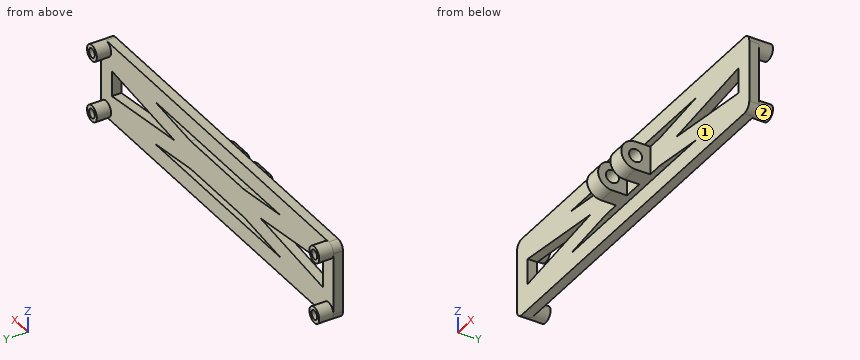
```python
from build123d import *

# Parameters (mm, degrees)
SKETCH2_W               = 80.1
SKETCH2_H               = 16.45
SKETCH2_W_2             = 72.76
SKETCH2_H_2             = 9.11
EXTRUDE_THIN1_DEPTH     = 2
EXTRUDE_THIN2_DEPTH     = 2
SKETCH6_W               = 18.3804486
SKETCH6_H               = 6
BOSS_EXTRUDE2_DEPTH     = 2
SKETCH7_R               = 1.375
BOSS_EXTRUDE3_DEPTH     = 3.8
LPATTERN1_COUNT         = 2
LPATTERN1_PITCH         = 8
FILLET2_R               = 1.69
SKETCH8_R               = 1.69
BOSS_EXTRUDE4_DEPTH     = 3
CUT_EXTRUDE1_START      = 3
SKETCH4_R               = 0.985
CUT_EXTRUDE1_DEPTH      = 4
MIRROR2_COPY_1_SKETCH_R = 1.69
MIRROR2_COPY_1_DEPTH    = 3
MIRROR2_START           = 3
MIRROR2_COPY_2_SKETCH_R = 0.985
MIRROR2_COPY_2_DEPTH    = 4


with BuildPart() as part:
    # Sketch2 → Extrude-Thin1 (new body)
    with BuildSketch(Plane(origin=(0, 0, 0), x_dir=(1, 0, 0), z_dir=(0, 1, 0))):
        Rectangle(SKETCH2_W, SKETCH2_H)
        Rectangle(SKETCH2_W_2, SKETCH2_H_2, mode=Mode.SUBTRACT)
    extrude(amount=EXTRUDE_THIN1_DEPTH)

    # Sketch3 → Extrude-Thin2 (add, through all)
    with BuildSketch(Plane(origin=(0, 2, 0), x_dir=(1, 0, 0), z_dir=(0, 1, 0))):
        Polygon((-36.607973326, 2.734216333), (36.152026674, -6.375783667), (36.607973326, -2.734216333), (-36.152026674, 6.375783667), align=None)
        Polygon((36.152026674, 6.375783667), (-36.607973326, -2.734216333), (-36.152026674, -6.375783667), (36.607973326, 2.734216333), align=None)
    extrude(amount=-EXTRUDE_THIN2_DEPTH)

    # Sketch6 → Boss-Extrude2 (add, through all)
    with BuildSketch(Plane(origin=(0, 2, 0), x_dir=(1, 0, 0), z_dir=(0, 1, 0))):
        Rectangle(SKETCH6_W, SKETCH6_H)
    extrude(amount=-BOSS_EXTRUDE2_DEPTH)

    # Sketch7 → Boss-Extrude3 (add)
    with BuildSketch(Plane(origin=(5.9, 0, 0), x_dir=(0, 0, -1), z_dir=(1, 0, 0))):
        with BuildLine():
            Line((-3, -3.1), (-3, 0))
            Line((-3, 0), (3, 0))
            Line((3, 0), (3, -3.1))
            ThreePointArc((3, -3.1), (0, -6.1), (-3, -3.1))
        make_face()
        with Locations((0, -3.1)):
            Circle(SKETCH7_R, mode=Mode.SUBTRACT)
    boss_extrude3 = extrude(amount=-BOSS_EXTRUDE3_DEPTH)

    # LPattern1: Boss-Extrude3 ×2
    with Locations(*[(-i * LPATTERN1_PITCH, 0, 0) for i in range(1, LPATTERN1_COUNT)]):
        add(boss_extrude3)

    # Fillet2
    fillet2_edges = [part.edges().sort_by_distance(p)[0] for p in [
        (40.05, 1, 8.225),
        (-40.05, 1, 8.225),
        (-40.05, 1, -8.225),
        (40.05, 1, -8.225),
    ]]
    fillet(fillet2_edges, radius=FILLET2_R)

    # Sketch8 → Boss-Extrude4 (add)
    with BuildSketch(Plane(origin=(0, 2, 0), x_dir=(1, 0, 0), z_dir=(0, 1, 0))):
        with Locations((-38.36, 6.535)):
            Circle(SKETCH8_R)
    boss_extrude4 = extrude(amount=BOSS_EXTRUDE4_DEPTH)

    # Sketch4 → Cut-Extrude1 (cut)
    with BuildSketch(Plane(origin=(0, 2, 0), x_dir=(1, 0, 0), z_dir=(0, 1, 0)).offset(CUT_EXTRUDE1_START)):
        with Locations((-38.36, 6.535)):
            Circle(SKETCH4_R)
    cut_extrude1 = extrude(amount=-CUT_EXTRUDE1_DEPTH, mode=Mode.SUBTRACT)

    # Mirror1: Boss-Extrude4, Cut-Extrude1 across plane
    add(boss_extrude4.mirror(Plane.XY))
    add(cut_extrude1.mirror(Plane.XY), mode=Mode.SUBTRACT)

    # Mirror2: Boss-Extrude4, Cut-Extrude1 across plane
    add(boss_extrude4.mirror(Plane(origin=(0, 0, 0), x_dir=(0, 0, 1), z_dir=(1, 0, 0))))
    add(cut_extrude1.mirror(Plane(origin=(0, 0, 0), x_dir=(0, 0, 1), z_dir=(1, 0, 0))), mode=Mode.SUBTRACT)

    # Mirror2 copy 1 sketch → Mirror2 copy 1 (add)
    with BuildSketch(Plane(origin=(0, 2, 0), x_dir=(-1, 0, 0), z_dir=(0, 1, 0))):
        with Locations((-38.36, 6.535)):
            Circle(MIRROR2_COPY_1_SKETCH_R)
    extrude(amount=MIRROR2_COPY_1_DEPTH)

    # Mirror2 copy 2 sketch → Mirror2 copy 2 (cut)
    with BuildSketch(Plane(origin=(0, 2, 0), x_dir=(-1, 0, 0), z_dir=(0, 1, 0)).offset(MIRROR2_START)):
        with Locations((-38.36, 6.535)):
            Circle(MIRROR2_COPY_2_SKETCH_R)
    extrude(amount=-MIRROR2_COPY_2_DEPTH, mode=Mode.SUBTRACT)


solid = part.part
```
The model under review builds one solid part; all positions refer to its coordinate system, in mm. Face numbers are marked on the shaded views. Coordinates: 2 decimals unless noted, no trailing zeros. Order: outer loops, then holes, each group sorted by start corner. A loop starts at its lowest first (then second) coordinate and runs counter-clockwise, first axis right, second up. Notation, with made-up numbers: M 1.5,50.5 L 44.5,50.5 A30 ccw 44.5,86.5 Z; hole C 45.25,13 d6. An arc over 180 degrees is marked long. One line per question, with ' | ' between items.
(1) Add section A-A, the plane y = 4. Write out the cut boundary in (x, z) (3 decimals).
Geometry results:
outline: C -38.36,-6.535 d3.38; C -38.36,6.535 d3.38; C 38.36,-6.535 d3.38; C 38.36,6.535 d3.38; hole C -38.36,-6.535 d1.97; hole C -38.36,6.535 d1.97; hole C 38.36,-6.535 d1.97; hole C 38.36,6.535 d1.97
(2) Insertion check: pin 1 (2 mm diameter, centred on x = 30, z = 2, fed in from +Y); pin 2 (1.6 mm diameter, centred on x = -38.36, z = -6.535, fed in from -Y); pin 3 (1.8 mm diameter, centred on y = -2.5, z = -0.5, fed in from +X); pin 4 (1.5 mm diameter, centred on x = -14.5, y = -1, fed in from -Z). Each pin has a flat end and moves straight along its axis. Give the tip position at first contact, or say it passes through.
Geometry results:
pin 1: stops at y = 2 | pin 2: stops at y = 0 | pin 3: stops at x = 5.9 | pin 4: passes through
(3) Add section B-B, the plane x = 31.5. Write out the cut boundary in (y, z) (3 decimals).
Geometry results:
outline: M 0,-8.225 L 2,-8.225 L 2,-2.095 L 0,-2.095 Z; M 0,2.095 L 2,2.095 L 2,8.225 L 0,8.225 Z
(4) For probe 1 along Z at (x, y) = (38.36, 3.3) (3 decimals); probe 2 along X at (y, z) = (-2, 2); probe 3 along Z at (x, y) = (-16, 1.5) (3 decimals), list the stretches that pass through material, from the lowest coordinate up. Write a range as from..to.
Geometry results:
probe 1: z = -8.225..-7.52, -5.55..-4.845, 4.845..5.55, 7.52..8.225 | probe 2: x = -5.9..-2.1, 2.1..5.9 | probe 3: z = -8.225..-4.555, -3.853..-0.154, 0.154..3.853, 4.555..8.225
(5) Add section C-C, the plane x = 16. Write out the cut boundary in (y, z) (3 decimals).
Geometry results:
outline: M 0,-8.225 L 2,-8.225 L 2,-4.555 L 0,-4.555 Z; M 0,-3.853 L 2,-3.853 L 2,-0.154 L 0,-0.154 Z; M 0,0.154 L 2,0.154 L 2,3.853 L 0,3.853 Z; M 0,4.555 L 2,4.555 L 2,8.225 L 0,8.225 Z
(6) The part is to be moulded in two halves that separate along X. For the marked faces 1 and 2, say which applies: +X half, -X half, draft (parallel to the pull), parting line (faces both ways), or undercut.
Geometry results:
face 1: draft | face 2: undercut
